Part model, mm, in its own coordinate system. A direction names the side the tool comes from. Give positions to 0.01 mm unless a question says otherwise; leave off trailing zeros. Order: outer loops, then holes, each group sorted by start corner. A loop starts at its lowest first (then second) coordinate and runs counter-clockwise, first axis right, second up. Notation, with made-up numbers: M -28,-9.75 L 6,-9.75 A20 cw 6,10.25 Z; hole C -7,67 d7. An arc over 180 degrees is marked long. Answer as a JSON object with one key per item and string values.
from build123d import *

# Parameters (mm, degrees)
BOSS_EXTRUDE1_DEPTH = 51.4
SKETCH2_R           = 1.5
CUT_EXTRUDE1_DEPTH  = 4.5
SKETCH3_R           = 11
BOSS_EXTRUDE2_DEPTH = 2.15
SKETCH5_R           = 4.725
CUT_EXTRUDE2_DEPTH  = 4
SKETCH4_R           = 2.5
BOSS_EXTRUDE3_DEPTH = 25.8
CUT_EXTRUDE3_START  = -15
CUT_EXTRUDE3_DEPTH  = 15
SKETCH7_W           = 25.7
SKETCH7_H           = 13.9
BOSS_EXTRUDE4_DEPTH = 7.1
FILLET1_R           = 1
FILLET2_R           = 2
CHAMFER1_SIZE       = 0.25


with BuildPart() as part:
    # Sketch1 → Boss-Extrude1 (new body)
    with BuildSketch(Plane.XY):
        Polygon((-21, 17), (-17, 21), (17, 21), (21, 17), (21, -17), (17, -21), (-17, -21), (-21, -17), align=None)
    extrude(amount=-BOSS_EXTRUDE1_DEPTH)

    # Sketch2 → Cut-Extrude1 (cut)
    with BuildSketch(Plane.XY):
        with Locations((-15.5, 15.5)):
            Circle(SKETCH2_R)
        with Locations(Location((15.5, 15.5, 0), (0, 0, 180))):
            Circle(SKETCH2_R)
        with Locations((15.5, -15.5)):
            Circle(SKETCH2_R)
        with Locations(Location((-15.5, -15.5, 0), (0, 0, 180))):
            Circle(SKETCH2_R)
    extrude(amount=-CUT_EXTRUDE1_DEPTH, mode=Mode.SUBTRACT)

    # Sketch3 → Boss-Extrude2 (add)
    with BuildSketch(Plane.XY):
        with Locations(Location((0, 0, 0), (0, 0, 180))):
            Circle(SKETCH3_R)
    extrude(amount=BOSS_EXTRUDE2_DEPTH)

    # Sketch5 → Cut-Extrude2 (cut)
    with BuildSketch(Plane.XY.offset(2.15)):
        Circle(SKETCH5_R)
    extrude(amount=-CUT_EXTRUDE2_DEPTH, mode=Mode.SUBTRACT)

    # Sketch4 → Boss-Extrude3 (add)
    with BuildSketch(Plane.XY.offset(-1.85)):
        Circle(SKETCH4_R)
    extrude(amount=BOSS_EXTRUDE3_DEPTH)

    # Sketch6 → Cut-Extrude3 (cut)
    with BuildSketch(Plane.XY.offset(23.95).offset(CUT_EXTRUDE3_START)):
        with BuildLine():
            Line((-1.5, 2), (1.5, 2))
            ThreePointArc((1.5, 2), (0, 2.5), (-1.5, 2))
        make_face()
    extrude(amount=CUT_EXTRUDE3_DEPTH, mode=Mode.SUBTRACT)

    # Sketch7 → Boss-Extrude4 (add)
    with BuildSketch(Plane(origin=(0, 0, -51.4), x_dir=(-1, 0, 0), z_dir=(0, 0, -1))):
        with Locations((0, 14.05)):
            Rectangle(SKETCH7_W, SKETCH7_H)
    extrude(amount=BOSS_EXTRUDE4_DEPTH)

    # Fillet1
    fillet1_edges = [part.edges().sort_by_distance(p)[0] for p in [
        (17, 21, -25.7),
        (21, 17, -25.7),
        (21, -17, -25.7),
        (17, -21, -25.7),
        (-17, -21, -25.7),
        (-21, -17, -25.7),
        (-21, 17, -25.7),
        (-17, 21, -25.7),
        (0, 7.1, -58.5),
        (-12.85, 14.05, -58.5),
        (0, 21, -58.5),
        (12.85, 14.05, -58.5),
    ]]
    fillet(fillet1_edges, radius=FILLET1_R)

    # Fillet2
    # the kernel refuses this fillet: 2 mm, written as the material it takes off along each edge
    with BuildSketch(Plane(origin=(-10.85, 19, -58.5), x_dir=(-1, 0, 0), z_dir=(0, -1, 0))) as fillet2_piece_1:
        with BuildLine():
            CenterArc((1, -1), 1, 0, 90)
            Line((2, -1), (2, 0))
            Line((2, 0), (1, 0))
        make_face()
    revolve(axis=Axis((-10.85, 19, -58.5), (0, 0, -1)), revolution_arc=90, mode=Mode.SUBTRACT)
    with BuildSketch(Plane(origin=(-10.85, 9.1, -58.5), x_dir=(0, -1, 0), z_dir=(1, 0, 0))) as fillet2_piece_2:
        with BuildLine():
            CenterArc((1, -1), 1, 0, 90)
            Line((2, -1), (2, 0))
            Line((2, 0), (1, 0))
        make_face()
    revolve(axis=Axis((-10.85, 9.1, -58.5), (0, 0, -1)), revolution_arc=90, mode=Mode.SUBTRACT)
    with BuildSketch(Plane(origin=(10.85, 19, -58.5), x_dir=(0, 1, 0), z_dir=(-1, 0, 0))) as fillet2_piece_3:
        with BuildLine():
            CenterArc((1, -1), 1, 0, 90)
            Line((2, -1), (2, 0))
            Line((2, 0), (1, 0))
        make_face()
    revolve(axis=Axis((10.85, 19, -58.5), (0, 0, -1)), revolution_arc=90, mode=Mode.SUBTRACT)
    with BuildSketch(Plane(origin=(10.85, 9.1, -58.5), x_dir=(1, 0, 0), z_dir=(0, 1, 0))) as fillet2_piece_4:
        with BuildLine():
            CenterArc((1, -1), 1, 0, 90)
            Line((2, -1), (2, 0))
            Line((2, 0), (1, 0))
        make_face()
    revolve(axis=Axis((10.85, 9.1, -58.5), (0, 0, -1)), revolution_arc=90, mode=Mode.SUBTRACT)
    with BuildSketch(Plane(origin=(12.85, 21, -51.4), x_dir=(-1, 0, 0), z_dir=(0, 0, -1))) as fillet2_piece_5:
        with BuildLine():
            CenterArc((FILLET2_R, -FILLET2_R), FILLET2_R, 90, 90)
            Line((0, -FILLET2_R), (0, 0))
            Line((0, 0), (FILLET2_R, 0))
        make_face()
    extrude(amount=7.1, mode=Mode.SUBTRACT)
    with BuildSketch(Plane(origin=(12.85, 7.1, -51.4), x_dir=(-1, 0, 0), z_dir=(0, 0, -1)), Plane(origin=(-12.85, 21, -51.4), x_dir=(1, 0, 0), z_dir=(0, 0, -1)), Plane(origin=(-12.85, 7.1, -51.4), x_dir=(0, 1, 0), z_dir=(0, 0, -1))) as fillet2_piece_6:
        with BuildLine():
            CenterArc((FILLET2_R, FILLET2_R), FILLET2_R, 180, 90)
            Line((0, FILLET2_R), (0, 0))
            Line((0, 0), (FILLET2_R, 0))
        make_face()
    extrude(amount=7.1, mode=Mode.SUBTRACT)

    # Chamfer1
    chamfer1_edges = [part.edges().sort_by_distance(p)[0] for p in [
        (16.96846987, 20.923879533, 0),
        (21, 0, -51.4),
        (19, -19, -51.4),
        (0, -21, -51.4),
        (-19, -19, -51.4),
        (-21, 0, -51.4),
        (-19, 19, -51.4),
        (-20.923879533, 16.96846987, -51.4),
        (-16.96846987, 20.923879533, -51.4),
        (-20.923879533, -16.96846987, -51.4),
        (-16.96846987, -20.923879533, -51.4),
        (16.96846987, -20.923879533, -51.4),
        (20.923879533, -16.96846987, -51.4),
        (20.923879533, 16.96846987, -51.4),
        (16.96846987, 20.923879533, -51.4),
        (-14, -15.5, 0),
        (14, -15.5, 0),
        (17, 15.5, 0),
        (-17, 15.5, 0),
        (11, 0, 0),
        (11, 0, 2.15),
        (-4.725, 0, 2.15),
        (-1.118033989, -2.236067977, 23.95),
        (0, 2, 23.95),
        (-13.717893219, 21, -51.4),
        (0, 21, 0),
        (13.717893219, 21, -51.4),
        (19, 19, 0),
        (19, 19, -51.4),
        (-19, 19, 0),
        (-21, 0, 0),
        (-19, -19, 0),
        (0, -21, 0),
        (19, -19, 0),
        (21, 0, 0),
        (-20.923879533, 16.96846987, 0),
        (-16.96846987, 20.923879533, 0),
        (-20.923879533, -16.96846987, 0),
        (-16.96846987, -20.923879533, 0),
        (16.96846987, -20.923879533, 0),
        (20.923879533, -16.96846987, 0),
        (20.923879533, 16.96846987, 0),
    ]]
    chamfer(chamfer1_edges, length=CHAMFER1_SIZE)


solid = part.part
1. Cut at C-C on z = -31.5. Give the cut face in (x, y).
Worked answers:
{"outline": "M -21,-16.59 A1 ccw -20.71,-17.29 L -17.29,-20.71 A1 ccw -16.59,-21 L 16.59,-21 A1 ccw 17.29,-20.71 L 20.71,-17.29 A1 ccw 21,-16.59 L 21,16.59 A1 ccw 20.71,17.29 L 17.29,20.71 A1 ccw 16.59,21 L -16.59,21 A1 ccw -17.29,20.71 L -20.71,17.29 A1 ccw -21,16.59 Z"}
2. Cut at D-D on y = 15.5. Give the cut face in (x, z), plus the area to 3 significant figures.
Worked answers:
{"outline": "M -21,-51.15 L -20.75,-51.4 L -12.85,-51.4 L -12.85,-57.5 A1 ccw -11.85,-58.5 L 11.85,-58.5 A1 ccw 12.85,-57.5 L 12.85,-51.4 L 20.75,-51.4 L 21,-51.15 L 21,-0.25 L 20.75,0 L 17.25,0 L 17,-0.25 L 17,-4.5 L 14,-4.5 L 14,-0.25 L 13.75,0 L -13.75,0 L -14,-0.25 L -14,-4.5 L -17,-4.5 L -17,-0.25 L -17.25,0 L -20.75,0 L -21,-0.25 Z", "area": "2,310 mm^2"}
3. Pin check, flat tips, straight feed: P1, Ø3, axis at y = 15, z = -55.5, coming from the +X side; P2, Ø5, axis at y = 14.5, z = -54, coming from the -X side; P3, Ø0.9, axis at x = -15, y = 15.5, coming from the +Z side. Stop position of each tip, or through.
Worked answers:
{"P1": "stops at x = 12.85", "P2": "stops at x = -12.85", "P3": "stops at z = -4.5"}
4. Two-plate mould, pull along X, no slides. Class faces 1 (the flat face through (18.89, 18.93, -0.12)), 2 (the cylindrical face through (4.507, 1.419, 0.051)), 3 (the cylindrical face through (-17, 15.57, -2.35)), 4 (the flat face through (0, -4, -51.4)): +X half, -X half, draft (parallel to the pull), parting line (faces both ways), or undercut.
Worked answers:
{"face 1": "+X half", "face 2": "undercut", "face 3": "undercut", "face 4": "draft"}
5. Cut at A-A on y = -15.5. Give the cut face in (x, z), plus the area to 3 significant figures.
Worked answers:
{"outline": "M -21,-51.15 L -20.75,-51.4 L 20.75,-51.4 L 21,-51.15 L 21,-0.25 L 20.75,0 L 17.25,0 L 17,-0.25 L 17,-4.5 L 14,-4.5 L 14,-0.25 L 13.75,0 L -13.75,0 L -14,-0.25 L -14,-4.5 L -17,-4.5 L -17,-0.25 L -17.25,0 L -20.75,0 L -21,-0.25 Z", "area": "2,130 mm^2"}
6. Which spindle directions (+Z, -Z, +X, -X, +Y, -Y) get a long thin tool onto all of the face, cutting with end or side? Do faces 5 (the flat face through (2, -2, -1.85)), 6 (the cylindrical face through (12.25, 20.43, -54.28)), 7 (the flat face through (-12.85, 14, -54)), 8 (the flat face through (18.94, -18.89, -51.27)). Say none if no direction does.
Worked answers:
{"face 5": "+Z", "face 6": "-Z, +X, +Y", "face 7": "-Z, -X, +Y, -Y", "face 8": "-Z, +X, -Y"}
7. Probe line 1 along Y through (x, z) = (-15.5, -2); line 2 along X through (y, z) = (15, -1); line 3 along Z through (x, y) = (-19, -7.5). List the from-to ranges inside material, lowest first.
Worked answers:
{"line 1": "y = -21 to -17, -14 to 14, 17 to 21", "line 2": "x = -21 to -16.91, -14.09 to 14.09, 16.91 to 21", "line 3": "z = -51.4 to 0"}
